```python
from build123d import *

# Parameters (mm, degrees)
SKETCH1_W            = 120
SKETCH1_H            = 80
PLATE_DEPTH          = 1
SLOT_CUT_DEPTH       = 73.117958928
SECOND_SLOT_COUNT    = 2
SECOND_SLOT_PITCH    = 13.38
MOTOR_OUTLINE_R      = 1.2
MOTOR_MOUNT_DEPTH    = 73.117958928
MOTORS_COUNT         = 3
MOTORS_PITCH         = 39
MOTORS_COUNT_DIR2    = 2
MOTORS_PITCH_DIR2    = 23
MOTOR_CUTOUT_DEPTH   = 73.117958928
CUTOUT_PATTERN_COUNT = 3
CUTOUT_PATTERN_PITCH = 39
FILLET1_R            = 10
CUT_EXTRUDE5_DEPTH   = 73.117958928
LPATTERN6_COUNT      = 2
LPATTERN6_PITCH      = 39


with BuildPart() as part:
    # Sketch1 → plate (new body)
    with BuildSketch(Plane.XY):
        Rectangle(SKETCH1_W, SKETCH1_H)
    extrude(amount=PLATE_DEPTH)

    # Sketch2 → slot_cut (cut, through all)
    with BuildSketch(Plane.XY.offset(1)):
        with BuildLine():
            Line((50, 26.8), (-50, 26.8))
            ThreePointArc((-50, 26.8), (-51.6, 28.4), (-50, 30))
            Line((-50, 30), (50, 30))
            ThreePointArc((50, 30), (51.6, 28.4), (50, 26.8))
        make_face()
    slot_cut = extrude(amount=-SLOT_CUT_DEPTH, mode=Mode.SUBTRACT)

    # second_slot: slot_cut ×2
    with Locations(*[(0, -i * SECOND_SLOT_PITCH, 0) for i in range(1, SECOND_SLOT_COUNT)]):
        add(slot_cut, mode=Mode.SUBTRACT)

    # motor_outline → motor_mount (cut, through all)
    with BuildSketch(Plane.XY.offset(1)):
        with Locations((-54, 6.42)):
            Circle(MOTOR_OUTLINE_R)
        with Locations(Location((-54, -9.58, 0), (0, 0, 180))):
            Circle(MOTOR_OUTLINE_R)
        with Locations((-24, -9.58)):
            Circle(MOTOR_OUTLINE_R)
        with Locations(Location((-24, 6.42, 0), (0, 0, 180))):
            Circle(MOTOR_OUTLINE_R)
    motor_mount = extrude(amount=-MOTOR_MOUNT_DEPTH, mode=Mode.SUBTRACT)

    # motors: motor_mount 3 × 2
    with Locations(*[(i * MOTORS_PITCH, -j * MOTORS_PITCH_DIR2, 0) for i in range(MOTORS_COUNT) for j in range(MOTORS_COUNT_DIR2) if (i, j) != (0, 0)]):
        add(motor_mount, mode=Mode.SUBTRACT)

    # motor_outline_5 → motor_cutout (cut, through all)
    with BuildSketch(Plane.XY.offset(1)):
        with BuildLine():
            Line((-26, -33), (-26, -11.58))
            Line((-26, -11.58), (-52, -11.58))
            Line((-52, -11.58), (-52, -33))
            ThreePointArc((-52, -33), (-50.535533906, -36.535533906), (-47, -38))
            Line((-47, -38), (-31, -38))
            ThreePointArc((-31, -38), (-27.464466094, -36.535533906), (-26, -33))
        make_face()
        with BuildLine():
            Line((-52, -11.58), (-26, -11.58))
            Line((-26, -11.58), (-26, 6.42))
            ThreePointArc((-26, 6.42), (-26.105468435, 7.441548218), (-26.417424305, 8.42))
            Line((-26.417424305, 8.42), (-51.582575695, 8.42))
            ThreePointArc((-51.582575695, 8.42), (-51.894531565, 7.441548218), (-52, 6.42))
            Line((-52, 6.42), (-52, -11.58))
        make_face()
        with BuildLine():
            Line((-51.582575695, 8.42), (-26.417424305, 8.42))
            ThreePointArc((-26.417424305, 8.42), (-28.261387212, 10.603300133), (-31, 11.42))
            Line((-31, 11.42), (-47, 11.42))
            ThreePointArc((-47, 11.42), (-49.738612788, 10.603300133), (-51.582575695, 8.42))
        make_face()
    motor_cutout = extrude(amount=-MOTOR_CUTOUT_DEPTH, mode=Mode.SUBTRACT)

    # cutout_pattern: motor_cutout ×3
    with Locations(*[(i * CUTOUT_PATTERN_PITCH, 0, 0) for i in range(1, CUTOUT_PATTERN_COUNT)]):
        add(motor_cutout, mode=Mode.SUBTRACT)

    # Fillet1
    fillet1_edges = [part.edges().sort_by_distance(p)[0] for p in [
        (-60, 40, 0.5),
        (60, 40, 0.5),
        (60, -40, 0.5),
        (-60, -40, 0.5),
    ]]
    fillet(fillet1_edges, radius=FILLET1_R)

    # Sketch4 → Cut-Extrude5 (cut, through all)
    with BuildSketch(Plane.XY.offset(1)):
        with BuildLine():
            Line((-17.5, 6.42), (-17.5, -32.58))
            ThreePointArc((-17.5, -32.58), (-19.5, -34.58), (-21.5, -32.58))
            Line((-21.5, -32.58), (-21.5, 6.42))
            ThreePointArc((-21.5, 6.42), (-19.5, 8.42), (-17.5, 6.42))
        make_face()
    cut_extrude5 = extrude(amount=-CUT_EXTRUDE5_DEPTH, mode=Mode.SUBTRACT)

    # LPattern6: Cut-Extrude5 ×2
    with Locations(*[(i * LPATTERN6_PITCH, 0, 0) for i in range(1, LPATTERN6_COUNT)]):
        add(cut_extrude5, mode=Mode.SUBTRACT)


solid = part.part
```
Build history of the part. All positions in model axes, mm. Give positions to 0.01 mm unless a question says otherwise; leave off trailing zeros. Loops run counter-clockwise (first coordinate to the right, second up) from the corner with the lowest first, then second, coordinate; pieces in that order, holes last. Notation, with made-up numbers: (-25, -11) -> (11, -11) arc R20 ccw to (11, 9) -> close; hole circle Ø6 at (72.25, -30). An arc over 180 degrees is marked (long way). One line per question, with ' | ' between items.
Q1. Cut at C-C, the plane x = 19.5. Write the cut outline in (y, z), plus the area to 3 significant figures.
Filled sheet:
outline: (-40, 0) -> (-34.58, 0) -> (-34.58, 1) -> (-40, 1) -> close; (8.42, 0) -> (13.42, 0) -> (13.42, 1) -> (8.42, 1) -> close; (16.62, 0) -> (26.8, 0) -> (26.8, 1) -> (16.62, 1) -> close; (30, 0) -> (40, 0) -> (40, 1) -> (30, 1) -> close | area: 30.6 mm²
Q2. Pull direction Y, two halves, no side cores. Call faces 1 (the cylindrical face through (56.99, 37.15, 0.51)), 2 (the flat face through (12.5, 9.4, 1)), 3 (the cylindrical face through (-52.855, -16.22, 0.507)): pulls with the +Y half, pulls with the -Y half, needs draft (parallel to the pull), parting line crosses it, or undercut.
Filled sheet:
face 1: pulls with the +Y half | face 2: needs draft | face 3: undercut
Q3. Cut at B-B, the plane y = -12.5. Write the cut outline in (x, z).
Filled sheet:
outline: (-60, 0) -> (-52, 0) -> (-52, 1) -> (-60, 1) -> close; (-26, 0) -> (-21.5, 0) -> (-21.5, 1) -> (-26, 1) -> close; (-17.5, 0) -> (-13, 0) -> (-13, 1) -> (-17.5, 1) -> close; (13, 0) -> (17.5, 0) -> (17.5, 1) -> (13, 1) -> close; (21.5, 0) -> (26, 0) -> (26, 1) -> (21.5, 1) -> close; (52, 0) -> (60, 0) -> (60, 1) -> (52, 1) -> close
Q4. Cut at D-D, the plane z = 0.3. Count the separate pieces of the cut face and the enclosed holes in it, plus the area to 3 significant figures.
Filled sheet:
separate pieces: 1 | enclosed holes: 31 | area: 4,620 mm²
Q5. Cut at A-A, the plane x = -15. Write the cut outline in (y, z).
Filled sheet:
outline: (-40, 0) -> (-33.78, 0) -> (-33.78, 1) -> (-40, 1) -> close; (-31.38, 0) -> (-17.78, 0) -> (-17.78, 1) -> (-31.38, 1) -> close; (-15.38, 0) -> (-10.78, 0) -> (-10.78, 1) -> (-15.38, 1) -> close; (-8.38, 0) -> (5.22, 0) -> (5.22, 1) -> (-8.38, 1) -> close; (7.62, 0) -> (13.42, 0) -> (13.42, 1) -> (7.62, 1) -> close; (16.62, 0) -> (26.8, 0) -> (26.8, 1) -> (16.62, 1) -> close; (30, 0) -> (40, 0) -> (40, 1) -> (30, 1) -> close
Q6. Drill centre lines: line 1 along Y through (x, z) = (-34, 0.4); line 2 along X through (y, z) = (-13, 0.7); line 3 along Y through (x, z) = (20, 0.1). Where is each one in solid material? Low to high. Write a range as [from, to].
Filled sheet:
line 1: y = [-40, -38], [11.42, 13.42], [16.62, 26.8], [30, 40] | line 2: x = [-60, -52], [-26, -21.5], [-17.5, -13], [13, 17.5], [21.5, 26], [52, 60] | line 3: y = [-40, -34.52], [8.36, 13.42], [16.62, 26.8], [30, 40]
